Read the model definition and answer for the solid it produces. Units are mm, in the model's axes. Coordinates: 2 decimals unless noted, no trailing zeros. Order: outer loops, then holes, each group sorted by start corner. A loop starts at its lowest first (then second) coordinate and runs counter-clockwise, first axis right, second up. Notation, with made-up numbers: (28, 70) -> (44, 70) arc R24 ccw to (44, 80) -> close; hole circle Ø9 at (36, 47.25). An arc over 180 degrees is marked (long way). Answer as a JSON object with one key per item and string values. Group by question number.
1) Consider L1, parallel to Y at x = -349, z = 0.15; L2, parallel to X at y = -213.5, z = 1.4. Determine where each line is inside the solid, lowest interval first.
2) Section A-A on z = 1.9 is taken. Determine the outline of the cut face in (x, y), and give its area (3 significant figures).
3) Section C-C on y = 233.5 is taken. Determine the outline of the cut face in (x, z), and give its area (3 significant figures).
4) Section B-B on x = -233.5 is taken. Determine the outline of the cut face in (y, z).
Autodesk Inventor part; units mm, degrees
ref_plane "YZ Plane" through (0, 0, 0) normal (1, 0, 0) x (0, 1, 0)
ref_plane "XZ Plane" through (0, 0, 0) normal (0, 1, 0) x (-1, 0, 0)
ref_plane "XY Plane" through (0, 0, 0) normal (0, 0, 1) x (1, 0, 0)
ref_plane "Work Plane1" through (0, 0, 0) normal (0, 0, 1) x (1, 0, 0)
sketch "Sketch1" plane through (0, 0, 0) normal (0, 0, 1) x (1, 0, 0)
  line L0 (-685.8, 266.7) -> (685.8, 266.7)
  line L1 (-685.8, -266.7) -> (-685.8, 266.7)
  line L2 (685.8, -266.7) -> (-685.8, -266.7)
  line L3 (685.8, 266.7) -> (685.8, -266.7)
  line L4 (-685.8, -266.7) -> (685.8, -266.7)
  line L5 (685.8, -266.7) -> (685.8, 266.7)
  line L6 (685.8, 266.7) -> (-685.8, 266.7)
  line L7 (-685.8, 266.7) -> (-685.8, -266.7)
  line L8 (-787.4, 368.3) -> (787.4, 368.3)
  line L9 (787.4, 368.3) -> (787.4, -368.3)
  line L10 (787.4, -368.3) -> (-787.4, -368.3)
  line L11 (-787.4, -368.3) -> (-787.4, 368.3)
  point P0 (0, 0)
  dimension "d0" = 101.6
extrude "Extrusion1" add sketch "Sketch1" along normal blind 2.54
properties part number "Reflective02" material "Polycarbonate, Clear"
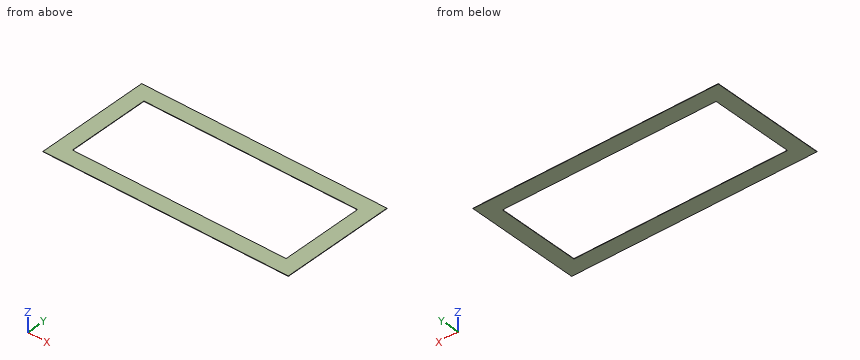
Worked answers:
{
 "1": {"L1": "y = -368.3 to -266.7, 266.7 to 368.3", "L2": "x = -787.4 to -685.8, 685.8 to 787.4"},
 "2": {"outline": "(-787.4, -368.3) -> (787.4, -368.3) -> (787.4, 368.3) -> (-787.4, 368.3) -> close; hole (-685.8, -266.7) -> (685.8, -266.7) -> (685.8, 266.7) -> (-685.8, 266.7) -> close", "area": "428,000 mm²"},
 "3": {"outline": "(-787.4, 0) -> (-685.8, 0) -> (-685.8, 2.54) -> (-787.4, 2.54) -> close; (685.8, 0) -> (787.4, 0) -> (787.4, 2.54) -> (685.8, 2.54) -> close", "area": "516 mm²"},
 "4": {"outline": "(-368.3, 0) -> (-266.7, 0) -> (-266.7, 2.54) -> (-368.3, 2.54) -> close; (266.7, 0) -> (368.3, 0) -> (368.3, 2.54) -> (266.7, 2.54) -> close"}
}
